Build history of the part. All positions in model axes, mm. Round coordinates to 2 decimals unless told otherwise and drop trailing zeros. Write each loop counter-clockwise with the first axis right and the second up, starting at its lowest first coordinate (ties: lowest second). Pieces come first, ordered by that corner, then holes. Notation, with made-up numbers: (5.25, 64.25) - (61.25, 64.25) arc R19 cw to (61.25, 91.25) - close; hole circle Ø2 at (-8.75, 82). An arc over 180 degrees is marked (long way). Write each question's results on one line, items separated by ' | '.
from build123d import *

# Parameters (mm, degrees)
SKETCH_1_R      = 1.5
EXTRUDE_1_DEPTH = 3


with BuildPart() as part:
    # ｽｹｯﾁ1 → ﾎﾞｽ - 押し出し1 (new body)
    with BuildSketch(Plane.XY):
        with BuildLine():
            Line((-3, 0), (-3, -30))
            ThreePointArc((-3, -30), (0, -33), (3, -30))
            Line((3, -30), (3, -12))
            Line((3, -12), (3, -8))
            Line((3, -8), (3, 0))
            ThreePointArc((3, 0), (0, 3), (-3, 0))
        make_face()
        Circle(SKETCH_1_R, mode=Mode.SUBTRACT)
        with Locations(Location((0, -30, 0), (0, 0, 180))):
            Circle(SKETCH_1_R, mode=Mode.SUBTRACT)
        with Locations((0, -13)):
            Circle(SKETCH_1_R, mode=Mode.SUBTRACT)
    extrude(amount=EXTRUDE_1_DEPTH)


solid = part.part
(1) Slice it at A-A, the plane z = 0.3. Write the cut outline in (x, y).
Worked answers:
outline: (-3, -30) arc R3 ccw to (3, -30) - (3, 0) arc R3 ccw to (-3, 0) - close; hole circle Ø3 at (0, -30); hole circle Ø3 at (0, -13); hole circle Ø3 at (0, 0)
(2) Slice it at C-C, the plane x = 0.65. Write the cut outline in (y, z).
Worked answers:
outline: (-32.93, 0) - (-31.35, 0) - (-31.35, 3) - (-32.93, 3) - close; (-28.65, 0) - (-14.35, 0) - (-14.35, 3) - (-28.65, 3) - close; (-11.65, 0) - (-1.35, 0) - (-1.35, 3) - (-11.65, 3) - close; (1.35, 0) - (2.93, 0) - (2.93, 3) - (1.35, 3) - close
(3) Flat gauge pin, fed straight in: pin 1 Ø2.5 at (x, y) = (0, -13) entering from -Z. Where does the tip first touch, or does it go through?
Worked answers:
pin 1: passes through
(4) Slice it at B-B, the plane y = -13. Write the cut outline in (x, z), and give its area (3 significant figures).
Worked answers:
outline: (-3, 0) - (-1.5, 0) - (-1.5, 3) - (-3, 3) - close; (1.5, 0) - (3, 0) - (3, 3) - (1.5, 3) - close | area: 9.00 mm2
(5) Drill centre lines: probe 1 along Y at (x, z) = (0, 2.1); probe 2 along X at (y, z) = (-30, 0.45); probe 3 along Y at (x, z) = (-0.95, 0.9). Where is each one in solid material? Low to high. Write a range as [from, to].
Worked answers:
probe 1: y = [-33, -31.5], [-28.5, -14.5], [-11.5, -1.5], [1.5, 3] | probe 2: x = [-3, -1.5], [1.5, 3] | probe 3: y = [-32.85, -31.16], [-28.84, -14.16], [-11.84, -1.16], [1.16, 2.85]
(6) Two-plate mould, pull along X, no slides. Class faces 1 (the cylindrical face through (0.195, -31.487, 1.479)), 2 (the flat face through (-3, -15, 1)), 3 (the flat face through (0, -15, 0)), 4 (the cylindrical face through (0, -33, 1)): released by +X, released by -X, zero draft, split by the parting line, or undercut.
Worked answers:
face 1: undercut | face 2: released by -X | face 3: zero draft | face 4: split by the parting line
